Autodesk Fusion 360 part; units mm, degrees
sketch "Sketch2" plane through (0, 0, 0) normal (0, 0, 1) x (1, 0, 0)
  line L0 (14.4655, -21) -> (-14.4655, -21)
  line L1 (-21, -14.4655) -> (-21, 14.4655)
  line L2 (1, 21) -> (14.4655, 21)
  line L3 (21, 14.4655) -> (21, -14.4655)
  line L4 (18.0312, -18.0312) -> (-18.0312, 18.0312) construction
  line L5 (-18.0312, -18.0312) -> (18.0312, 18.0312) construction
  arc A0 (21, 14.4655) -> (14.4655, 21) centre (0, 0) ccw
  arc A1 (-21, -14.4655) -> (-14.4655, -21) centre (0, 0) ccw
  arc A2 (14.4655, -21) -> (21, -14.4655) centre (0, 0) ccw
  line L6 (-21, 14.4655) -> (-21, 21)
  line L7 (0.0943, 21.9057) -> (0.0943, 41)
  line L8 (0.0943, 41) -> (-21, 41)
  line L9 (-21, 41) -> (-21, 21)
  line L10 (0.0943, 21.9057) -> (1, 21)
  line L11 (-24.5, 38.866) -> (-24.5, 21)
  line L12 (-24.5, 14.4655) -> (-24.5, 21)
  line L13 (-24.5, -15.5161) -> (-24.5, 14.4655)
  arc A3 (-24.5, -15.5161) -> (-15.5161, -24.5) centre (0, 0) ccw
  line L14 (15.5161, -24.5) -> (-15.5161, -24.5)
  arc A4 (15.5161, -24.5) -> (24.5, -15.5161) centre (0, 0) ccw
  line L15 (24.5, 15.5161) -> (24.5, -15.5161)
  arc A5 (24.5, 15.5161) -> (15.5161, 24.5) centre (0, 0) ccw
  line L16 (3.5, 24.5) -> (15.5161, 24.5)
  line L17 (3.5, 24.5) -> (3.5, 38.9603)
  line L18 (-24.5, 38.866) -> (-21, 38.866)
  line L19 (0.0943, 38.9603) -> (3.5, 38.9603)
  dimension "d3" = 51
  dimension "d6" = 20
extrude "Extrude9" add sketch "Sketch2" along normal blind 17 contours L0 L1 L2 L3 A0 A1 A2 L6 L7 L9 L10 L11 L12 L13 A3 L14 A4 L15 A5 L16 L17 L18 L19
sketch "Sketch7" plane through (-24.5, 0, 0) normal (-1, 0, 0) x (0, 0, 1)
  line L0 (0, 38.866) -> (0, -15.5161)
  line L1 (0, -15.5161) -> (17, -15.5161)
  line L2 (17, -15.5161) -> (17, 38.866)
  line L3 (17, 38.866) -> (0, 38.866)
sketch "Sketch8" plane through (3.5, 0, 0) normal (1, 0, 0) x (0, 0, -1)
  line L0 (0, 24.5) -> (0, 38.9603)
  line L1 (0, 38.9603) -> (-17, 38.9603)
  line L2 (-17, 38.9603) -> (-17, 24.5)
  line L3 (-17, 24.5) -> (0, 24.5)
  circle A0 centre (-8.5, 31) radius 2.7
  dimension "d32" = 5.4
extrude "Extrude10" cut sketch "Sketch8" against normal blind 50 contours A0
sketch "Sketch9" plane through (3.5, 0, 0) normal (1, 0, 0) x (0, 0, -1)
  circle A0 centre (-8.5, 31) radius 2.7
  line L0 (0, 24.5) -> (0, 38.9603)
  line L1 (0, 38.9603) -> (-17, 38.9603)
  line L2 (-17, 38.9603) -> (-17, 24.5)
  line L3 (-17, 24.5) -> (0, 24.5)
  circle A1 centre (-8.5, 31) radius 5
  dimension "d35" = 10
extrude "Extrude11" cut sketch "Sketch9" against normal blind 0.5 contours A1
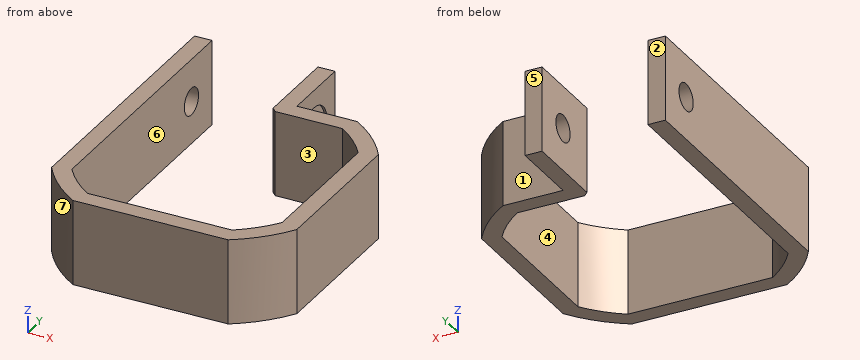
Could you check a few things on this model? Use its own coordinates, in mm. Face numbers are marked on the shaded views. A direction names the side the tool comes from. Give positions to 0.01 mm unless a question says otherwise; leave off trailing zeros. Order: outer loops, then holes, each group sorted by start corner. A loop starts at its lowest first (then second) coordinate and runs counter-clockwise, first axis right, second up. Notation, with made-up numbers: (76, 9) -> (112, 9) arc R23 ccw to (112, 32) -> close; hole circle Ø9 at (3.25, -13.5). An arc over 180 degrees is marked (long way). Return JSON: item names as keys, results as strings.
1. Imagine slicing it at A-A on y = 31. List the corners of the cut face in (x, z) for me, then the cut area to 3 significant figures.
Answer list:
{"outline": "(-24.5, 0) -> (-21, 0) -> (-21, 5.8) -> (-24.5, 5.8) -> close; (-24.5, 11.2) -> (-21, 11.2) -> (-21, 17) -> (-24.5, 17) -> close; (0.09, 0) -> (3.5, 0) -> (3.5, 3.5) -> (3, 3.5) -> (3, 5.8) -> (0.09, 5.8) -> close; (0.09, 11.2) -> (3, 11.2) -> (3, 13.5) -> (3.5, 13.5) -> (3.5, 17) -> (0.09, 17) -> close", "area": "77.8 mm2"}
2. For pin 1 Ø4.5 at (y, z) = (30, 8) entering from +X; pin 2 Ø1 at (x, z) = (-22, 6.5) entering from +Y; pin 3 Ø1 at (x, z) = (17, 15) entering from -Y, each with a flat end and sliding along its axis, tell me the tip position at first contact or that it passes through.
Answer list:
{"pin 1": "stops at x = 3", "pin 2": "stops at y = 38.87", "pin 3": "stops at y = -23.85"}
3. Thinking about a two-plate mould opening in Y: for the marked faces 4, 5, 6 and 7, which applies, pulls with the +Y half, pulls with the -Y half, needs draft (parallel to the pull), parting line crosses it, or undercut?
Answer list:
{"face 4": "undercut", "face 5": "pulls with the +Y half", "face 6": "needs draft", "face 7": "pulls with the -Y half"}
4. Imagine slicing it at D-D on x = 18.5. List the corners of the cut face in (y, z) for me.
Answer list:
{"outline": "(-22.33, 0) -> (-17.55, 0) -> (-17.55, 17) -> (-22.33, 17) -> close; (17.55, 0) -> (22.33, 0) -> (22.33, 17) -> (17.55, 17) -> close"}
5. Imagine slicing it at B-B on y = 7.5. List the corners of the cut face in (x, z) for me, then the cut area to 3 significant figures.
Answer list:
{"outline": "(-24.5, 0) -> (-21, 0) -> (-21, 17) -> (-24.5, 17) -> close; (21, 0) -> (24.5, 0) -> (24.5, 17) -> (21, 17) -> close", "area": "119 mm2"}
6. I need wall thicknesses on line 1 (X direction, y = 28, z = 8.75); line 2 (X direction, y = 2, z = 16); line 3 (Y direction, x = 2.1, z = 8.5). Which ranges of each line are inside material? Lowest first, please. Write a range as from..to.
Answer list:
{"line 1": "x = -24.5..-21, 0.09..3", "line 2": "x = -24.5..-21, 21..24.5", "line 3": "y = -24.5..-21, 21..28.3, 33.7..38.96"}
7. On a 3-axis mill with a long thin cutter (end or side, diameter ignored), from which of +Z, -Z, +X, -X, +Y, -Y can I reach the whole of each face in a straight line? I mean the marked faces 1, 2 and 3. Say none if no direction works.
Answer list:
{"face 1": "+Z, -Z, +X, +Y", "face 2": "+Z, -Z, -X, +Y", "face 3": "+Z, -Z"}
8. Imagine slicing it at C-C on z = 8.5. Give the number of separate pieces and of enclosed holes in the cut face, then the cut area to 3 significant figures.
Answer list:
{"separate pieces": "3", "enclosed holes": "0", "area": "576 mm2"}
